from build123d import *
from build123d.topology import SkipClean

# Parameters (mm, degrees)
BASPROSKE_W         = 2
BASPROSKE_H         = 8.25
TOOTHCUT_DEPTH      = 12.837440602
TEETHCUTS_COUNT     = 10
TEETHCUTS_ANGLE     = 324
BORSKE_R            = 2.5
BORE_DEPTH          = 50.0000508
SKETCH1_R           = 2.5
SKETCH1_R_2         = 1.4
BOSS_EXTRUDE1_DEPTH = 2
SKETCH2_R           = 2.8
SKETCH2_R_2         = 1.6
BOSS_EXTRUDE2_DEPTH = 1
CHAMFER1_SIZE       = 1.5
SKETCH3_R           = 1.5
BOSS_EXTRUDE3_DEPTH = 1
SKETCH4_R           = 1.6
SKETCH4_R_2         = 1.4
BOSS_EXTRUDE4_DEPTH = 1
BOSS_EXTRUDE5_START = 1
SKETCH5_R           = 1.5
SKETCH5_R_2         = 1.4
BOSS_EXTRUDE5_DEPTH = 1


with BuildPart() as part:
    # BasProSke → Base-Revolve (revolve)
    with BuildSketch(Plane(origin=(0, 0, 0), x_dir=(1, 0, 0), z_dir=(0, 1, 0)), mode=Mode.PRIVATE) as base_revolve_sk:
        with Locations((1, 4.125)):
            Rectangle(BASPROSKE_W, BASPROSKE_H)
    revolve(base_revolve_sk.sketch.rotate(Axis((-10, 0, 0), (1, 0, 0)), 180), axis=Axis((-10, 0, 0), (1, 0, 0)))

    # TooCutSke → ToothCut (cut, through all)
    with BuildSketch(Plane(origin=(0, 0, 0), x_dir=(0, 0, -1), z_dir=(1, 0, 0))):
        with BuildLine():
            ThreePointArc((0.810777273, 5.091094458), (0, 5.15525), (-0.810777273, 5.091094458))
            ThreePointArc((-0.810777273, 5.091094458), (-1.154893166, 6.765492881), (-2.421785774, 7.913102983))
            ThreePointArc((-2.421785774, 7.913102983), (0, 8.2754), (2.421785774, 7.913102983))
            ThreePointArc((2.421785774, 7.913102983), (1.154893166, 6.765492881), (0.810777273, 5.091094458))
        make_face()
    toothcut = extrude(amount=TOOTHCUT_DEPTH, mode=Mode.SUBTRACT)

    # TeethCuts: ToothCut ×10 about axis
    teethcuts_axis = Axis((-10, 0, 0), (1, 0, 0))
    for i in range(1, TEETHCUTS_COUNT):
        add(toothcut.rotate(teethcuts_axis, i * TEETHCUTS_ANGLE / (TEETHCUTS_COUNT - 1)), mode=Mode.SUBTRACT)

    # BorSke → Bore (cut, symmetric)
    with BuildSketch(Plane(origin=(0, 0, 0), x_dir=(0, 0, -1), z_dir=(1, 0, 0))):
        with Locations(Location((0, 0, 0), (0, 0, 180))):
            Circle(BORSKE_R)
    extrude(amount=BORE_DEPTH, both=True, mode=Mode.SUBTRACT)

    # Sketch1 → Boss-Extrude1 (add)
    with BuildSketch(Plane(origin=(2, 0, 0), x_dir=(0, 0, -1), z_dir=(1, 0, 0))):
        Circle(SKETCH1_R)
        Circle(SKETCH1_R_2, mode=Mode.SUBTRACT)
    extrude(amount=-BOSS_EXTRUDE1_DEPTH)

    # Sketch2 → Boss-Extrude2 (add)
    with BuildSketch(Plane.ZY):
        with Locations(Location((0, 0, 0), (0, 0, 180))):
            Circle(SKETCH2_R)
        Circle(SKETCH2_R_2, mode=Mode.SUBTRACT)
    extrude(amount=BOSS_EXTRUDE2_DEPTH)

    # Chamfer1
    # the kernel refuses this chamfer: 1.5 mm, written as the material it adds along each edge
    with BuildSketch(Plane(origin=(0, 0, 0), x_dir=(0, 0, -1), z_dir=(0, 1, 0))) as chamfer1_piece_1_section:
        Polygon((2.8 + CHAMFER1_SIZE, 0), (2.8, CHAMFER1_SIZE), (2.8, 0), align=None)
    chamfer1_piece_1 = revolve(axis=Axis((0, 0, 0), (-1, 0, 0)), mode=Mode.PRIVATE)
    chamfer1_piece_1 = split(chamfer1_piece_1, bisect_by=Plane(origin=(-1, 0, 3.801160136), z_dir=(1, 0, 0)), keep=Keep.TOP, mode=Mode.PRIVATE)
    add(chamfer1_piece_1)

    # Sketch3 → Boss-Extrude3 (add)
    with SkipClean():  # the faces are left unmerged after this step: merging them gives an invalid solid
        with BuildSketch(Plane(origin=(2, 0, 0), x_dir=(0, 0, -1), z_dir=(1, 0, 0))):
            with BuildLine():
                ThreePointArc((8.248240616, 0.170372351), (6.772423309, 0.99612057), (5.092462515, 0.802139699))
                ThreePointArc((5.092462515, 0.802139699), (4.902934106, 1.59305986), (4.591374603, 2.344329716))
                ThreePointArc((4.591374603, 2.344329716), (6.06451053, 3.174852073), (6.773109188, 4.710360064))
                ThreePointArc((6.773109188, 4.710360064), (6.674390204, 4.849228331), (6.572824477, 4.986028319))
                ThreePointArc((6.572824477, 4.986028319), (4.893500569, 4.786609013), (3.648402832, 3.642219012))
                ThreePointArc((3.648402832, 3.642219012), (3.030179922, 4.17068486), (2.336537648, 4.59534486))
                ThreePointArc((2.336537648, 4.59534486), (3.040160855, 6.133139134), (2.710880259, 7.791895034))
                ThreePointArc((2.710880259, 7.791895034), (2.549390204, 7.846216259), (2.386812789, 7.897190938))
                ThreePointArc((2.386812789, 7.897190938), (1.145426936, 6.748775503), (0.810777273, 5.091094458))
                ThreePointArc((0.810777273, 5.091094458), (0, 5.15525), (-0.810777273, 5.091094458))
                ThreePointArc((-0.810777273, 5.091094458), (-1.145426936, 6.748775503), (-2.386812789, 7.897190938))
                ThreePointArc((-2.386812789, 7.897190938), (-2.549390204, 7.846216259), (-2.710880259, 7.791895034))
                ThreePointArc((-2.710880259, 7.791895034), (-3.040160855, 6.133139134), (-2.336537648, 4.59534486))
                ThreePointArc((-2.336537648, 4.59534486), (-3.030179922, 4.17068486), (-3.648402832, 3.642219012))
                ThreePointArc((-3.648402832, 3.642219012), (-4.893500569, 4.786609013), (-6.572824477, 4.986028319))
                ThreePointArc((-6.572824477, 4.986028319), (-6.674390204, 4.849228331), (-6.773109188, 4.710360064))
                ThreePointArc((-6.773109188, 4.710360064), (-6.06451053, 3.174852073), (-4.591374603, 2.344329716))
                ThreePointArc((-4.591374603, 2.344329716), (-4.902934106, 1.59305986), (-5.092462515, 0.802139699))
                ThreePointArc((-5.092462515, 0.802139699), (-6.772423309, 0.99612057), (-8.248240616, 0.170372351))
                ThreePointArc((-8.248240616, 0.170372351), (-8.25, 0), (-8.248240616, -0.170372351))
                ThreePointArc((-8.248240616, -0.170372351), (-6.772423309, -0.99612057), (-5.092462515, -0.802139699))
                ThreePointArc((-5.092462515, -0.802139699), (-4.902934106, -1.59305986), (-4.591374603, -2.344329716))
                ThreePointArc((-4.591374603, -2.344329716), (-6.06451053, -3.174852073), (-6.773109188, -4.710360064))
                ThreePointArc((-6.773109188, -4.710360064), (-6.674390204, -4.849228331), (-6.572824477, -4.986028319))
                ThreePointArc((-6.572824477, -4.986028319), (-4.893500569, -4.786609013), (-3.648402832, -3.642219012))
                ThreePointArc((-3.648402832, -3.642219012), (-3.030179922, -4.17068486), (-2.336537648, -4.59534486))
                ThreePointArc((-2.336537648, -4.59534486), (-3.040160855, -6.133139134), (-2.710880259, -7.791895034))
                ThreePointArc((-2.710880259, -7.791895034), (-2.549390204, -7.846216259), (-2.386812789, -7.897190938))
                ThreePointArc((-2.386812789, -7.897190938), (-1.145426936, -6.748775503), (-0.810777273, -5.091094458))
                ThreePointArc((-0.810777273, -5.091094458), (0, -5.15525), (0.810777273, -5.091094458))
                ThreePointArc((0.810777273, -5.091094458), (1.145426936, -6.748775503), (2.386812789, -7.897190938))
                ThreePointArc((2.386812789, -7.897190938), (2.549390204, -7.846216259), (2.710880259, -7.791895034))
                ThreePointArc((2.710880259, -7.791895034), (3.040160855, -6.133139134), (2.336537648, -4.59534486))
                ThreePointArc((2.336537648, -4.59534486), (3.030179922, -4.17068486), (3.648402832, -3.642219012))
                ThreePointArc((3.648402832, -3.642219012), (4.893500569, -4.786609013), (6.572824477, -4.986028319))
                ThreePointArc((6.572824477, -4.986028319), (6.674390204, -4.849228331), (6.773109188, -4.710360064))
                ThreePointArc((6.773109188, -4.710360064), (6.06451053, -3.174852073), (4.591374603, -2.344329716))
                ThreePointArc((4.591374603, -2.344329716), (4.902934106, -1.59305986), (5.092462515, -0.802139699))
                ThreePointArc((5.092462515, -0.802139699), (6.772423309, -0.99612057), (8.248240616, -0.170372351))
                ThreePointArc((8.248240616, -0.170372351), (8.25, 0), (8.248240616, 0.170372351))
            make_face()
            Circle(SKETCH3_R, mode=Mode.SUBTRACT)
        extrude(amount=BOSS_EXTRUDE3_DEPTH)

    # Sketch4 → Boss-Extrude4 (add)
    with SkipClean():  # the faces are left unmerged after this step: merging them gives an invalid solid
        with BuildSketch(Plane.ZY):
            Circle(SKETCH4_R)
            with Locations(Location((0, 0, 0), (0, 0, 180))):
                Circle(SKETCH4_R_2, mode=Mode.SUBTRACT)
        extrude(amount=BOSS_EXTRUDE4_DEPTH)

    # Sketch5 → Boss-Extrude5 (add)
    with SkipClean():  # the faces are left unmerged after this step: merging them gives an invalid solid
        with BuildSketch(Plane(origin=(2, 0, 0), x_dir=(0, 0, -1), z_dir=(1, 0, 0)).offset(BOSS_EXTRUDE5_START)):
            Circle(SKETCH5_R)
            Circle(SKETCH5_R_2, mode=Mode.SUBTRACT)
        extrude(amount=-BOSS_EXTRUDE5_DEPTH)


solid = part.part
Geometry check sheet. Reference: the model listing, model coordinates, mm. Round coordinates to 2 decimals unless told otherwise and drop trailing zeros. Loops run counter-clockwise (first coordinate to the right, second up) from the corner with the lowest first, then second, coordinate; pieces in that order, holes last.
Item 1: Cross-section at A-A on z = 0. Record the boundary of the cut face in (x, y).
Item 2: Cross-section at C-C on x = -0.4. Record the boundary of the cut face in (y, z).
Item 3: Gauge pin test, flat end, axial feed: pin 1 (1 mm diameter, centred on x = 0.5, y = -4, fed in from +Z). Record the tip position at first contact, or that the pin passes through.
Item 4: Cross-section at D-D on y = 5.75. Record the boundary of the cut face in (x, z).
Item 5: Cross-section at B-B on z = -6. Record the boundary of the cut face in (x, y), then the cut area to 3 significant figures.
Item 6: Thickness scan on line 1 (Y direction, x = 0.7, z = -2.5); line 2 (Z direction, x = 2.3, y = -4.25); line 3 (Y direction, x = 1.45, z = 0). Record the ranges inside material, lowest first.
Answer sheet:
1. outline: (-1, -3.3) - (0, -4.3) - (0, -5.16) - (3, -5.16) - (3, -1.4) - (-1, -1.4) - close; (-1, 1.4) - (3, 1.4) - (3, 5.16) - (0, 5.16) - (0, 4.3) - (-1, 3.3) - close
2. outline: circle Ø7.8 at (0, 0); hole circle Ø2.8 at (0, 0)
3. pin 1: stops at z = 6.74
4. outline: (0, -2.97) - (3, -2.97) - (3, -0.82) - (0, -0.82) - close; (0, 0.82) - (3, 0.82) - (3, 2.97) - (0, 2.97) - close
5. outline: (0, -5.04) - (3, -5.04) - (3, -3.11) - (0, -3.11) - close; (0, -1.04) - (3, -1.04) - (3, 1.04) - (0, 1.04) - close; (0, 3.11) - (3, 3.11) - (3, 5.04) - (0, 5.04) - close
5. area: 17.8 mm2
6. line 1: y = -7.86 to -4.79, -4.51 to 4.51, 4.79 to 7.86
6. line 2: z = -6.68 to -4.12, -2.92 to 2.92, 4.12 to 6.68
6. line 3: y = -5.16 to -1.4, 1.4 to 5.16
